from build123d import *

# Parameters (mm, degrees)
F0_W     = 90
F0_H     = 35
F1_DEPTH = 10
F3_R     = 3
F4_DEPTH = 10.001
F5_D     = 6.3
F5_DEPTH = 20
F5_TIP   = 1.8927109499


with BuildPart() as f1:
    # F0 (on Front) → F1 (new body)
    with BuildSketch(Plane.XZ):
        Rectangle(F0_W, F0_H)
    extrude(amount=F1_DEPTH)

    # F3 (on face) → F4 (cut, through all)
    with BuildSketch(Plane.XZ.offset(10)):
        with Locations((-37.5, 10)):
            Circle(F3_R)
        with Locations((-37.5, -10)):
            Circle(F3_R)
        with Locations((37.5, -10)):
            Circle(F3_R)
        with Locations((37.5, 10)):
            Circle(F3_R)
    extrude(amount=-F4_DEPTH, mode=Mode.SUBTRACT)

    # F5
    with Locations(Plane.XZ.offset(10)):
        with Locations((-23, 6.5), (-23, -6.5), (23, -6.5), (23, 6.5)):
            Hole(F5_D / 2, depth=F5_DEPTH)
            with Locations((0, 0, -(F5_DEPTH + F5_TIP / 2))):  # 118° drill point
                Cone(0, F5_D / 2, F5_TIP, mode=Mode.SUBTRACT)


solid = f1.part
Input: part model. Units: mm. Frame: model coordinates. Coordinates: 2 decimals unless noted, no trailing zeros. Order: outer loops, then holes, each group sorted by start corner. A loop starts at its lowest first (then second) coordinate and runs counter-clockwise, first axis right, second up. Notation, with made-up numbers: M 4.25,19 L 43.25,19 A19 ccw 43.25,55 Z; hole C 71,2 d8. An arc over 180 degrees is marked long. Write item = value, one per line. Start each with the question number.
(1) Pull-direction query (Z, two-part tool) for faces 1 (the flat face through (-1, -10, 0)), 2 (the cylindrical face through (-40.5, -5.1, 10.1)), 3 (the flat face through (-1, -5, 17.5)); classes: released by +Z, released by -Z, zero draft, split by the parting line, or undercut.
(2) Line query: line 1 along Z through (x, y) = (-37.5, -5.5); line 2 along Z through (x, y) = (23, -6.75); line 3 along X through (y, z) = (-1.25, -9). Output: solid intervals per line, ascending. Write a range as [from, to].
(3) Section C-C on z = 11.5. Output: boundary loops of the cut face in (x, y).
(4) Section A-A on x = -23. Output: boundary loops of the cut face in (y, z).
(5) Section B-B on y = -3. Give the number of separate pieces and of enclosed holes in the cut face, and give its area (3 significant figures).
Result set:
q1.face_1 = zero draft
q1.face_2 = undercut
q1.face_3 = released by +Z
q2.line_1 = [-17.5, -13], [-7, 7], [13, 17.5]
q2.line_2 = [-17.5, -9.65], [-3.35, 3.35], [9.65, 17.5]
q2.line_3 = [-45, -40.33], [-34.67, -24.92], [-21.08, 21.08], [24.92, 34.67], [40.33, 45]
q3.outline = M -45,-10 L -40.1,-10 L -40.1,0 L -45,0 Z; M -34.9,-10 L 34.9,-10 L 34.9,0 L -34.9,0 Z; M 40.1,-10 L 45,-10 L 45,0 L 40.1,0 Z
q4.outline = M -10,-17.5 L 0,-17.5 L 0,-9.65 L -10,-9.65 Z; M -10,-3.35 L 0,-3.35 L 0,3.35 L -10,3.35 Z; M -10,9.65 L 0,9.65 L 0,17.5 L -10,17.5 Z
q5.separate_pieces = 1
q5.enclosed_holes = 8
q5.area = 2,910 mm²
